Can you work these out from the model? Positions are in its coordinate system, mm. A direction names the side the tool comes from. Round coordinates to 2 decimals unless told otherwise and drop trailing zeros. Order: outer loops, then holes, each group sorted by start corner. A loop starts at its lowest first (then second) coordinate and runs counter-clockwise, first axis right, second up.
from build123d import *

# Parameters (mm, degrees)
SKETCH_1_W          = 21
SKETCH_1_H          = 34
EXTRUDE_1_DEPTH     = 9
SKETCH_4_W          = 21
SKETCH_4_H          = 10
CUT_EXTRUDE_1_DEPTH = 6
SKETCH_5_W          = 21
SKETCH_5_H          = 15
CUT_EXTRUDE_2_DEPTH = 3
SKETCH_6_W          = 13.003696042
SKETCH_6_H          = 17
CUT_EXTRUDE_3_DEPTH = 22.914607001
CUT_EXTRUDE_4_DEPTH = 1.8
CUT_EXTRUDE_5_REACH = 29.178
SKETCH_11_R         = 1.65
HOLE_WIZARD_1_D     = 1.3


with BuildPart() as part:
    # 草图1 → 凸台-拉伸1 (new body)
    with BuildSketch(Plane(origin=(0, 0, 0), x_dir=(1, 0, 0), z_dir=(0, 1, 0))):
        Rectangle(SKETCH_1_W, SKETCH_1_H)
    extrude(amount=EXTRUDE_1_DEPTH)

    # 草图4 → 切除-拉伸1 (cut)
    with BuildSketch(Plane.XZ):
        with Locations((0, -12)):
            Rectangle(SKETCH_4_W, SKETCH_4_H)
    extrude(amount=-CUT_EXTRUDE_1_DEPTH, mode=Mode.SUBTRACT)

    # 草图5 → 切除-拉伸2 (cut)
    with BuildSketch(Plane.XZ):
        with Locations((0, -9.5)):
            Rectangle(SKETCH_5_W, SKETCH_5_H)
    extrude(amount=-CUT_EXTRUDE_2_DEPTH, mode=Mode.SUBTRACT)

    # 草图6 → 切除-拉伸3 (cut, through all)
    with BuildSketch(Plane(origin=(0, 9, 0), x_dir=(1, 0, 0), z_dir=(0, 1, 0))):
        with Locations((0, -8.5)):
            Rectangle(SKETCH_6_W, SKETCH_6_H)
    extrude(amount=-CUT_EXTRUDE_3_DEPTH, mode=Mode.SUBTRACT)

    # 草图9 → M3 六角圆柱头螺钉的柱形沉头孔1 (revolve, cut)
    with BuildSketch(Plane(origin=(10.5, 4.5, 11.5), x_dir=(0, 0, -1), z_dir=(0, 1, 0))):
        Polygon((0, 0), (0, 3.998151979), (1.7, 3.998151979), (1.7, 3.4), (3, 3.4), (3, 0.025), (3.025, 0), align=None)
    revolve(axis=Axis((16.85, 4.5, 11.5), (-1, 0, 0)), mode=Mode.SUBTRACT)

    # 草图10 → 切除-拉伸4 (cut)
    with BuildSketch(Plane.ZY.offset(10.5)):
        Polygon((13.174315781, 1.6), (14.848631561, 4.5), (13.174315781, 7.4), (9.825684219, 7.4), (8.151368439, 4.5), (9.825684219, 1.6), align=None)
    extrude(amount=-CUT_EXTRUDE_4_DEPTH, mode=Mode.SUBTRACT)

    # 草图11 → 切除-拉伸5 (cut, up to next)
    with BuildSketch(Plane.ZY.offset(8.7), mode=Mode.PRIVATE) as cut_extrude_5_sk1:
        with Locations((11.5, 4.5)):
            Circle(SKETCH_11_R)
    cut_extrude_5_tool1 = extrude(cut_extrude_5_sk1.sketch, amount=-CUT_EXTRUDE_5_REACH, mode=Mode.PRIVATE) & part.part
    add(cut_extrude_5_tool1.solids().sort_by_distance((-8.7, 4.5, 11.5))[0], mode=Mode.SUBTRACT)

    # 孔1 (through all)
    with Locations(Plane(origin=(0, 9, 0), x_dir=(1, 0, 0), z_dir=(0, 1, 0))):
        with Locations((-7.5, 4.5), (7.5, 4.5)):
            Hole(HOLE_WIZARD_1_D / 2)


solid = part.part
(1) I want a section at B-B, the plane z = 11.5. List the corners of the cut face in (x, y) for me (3 decimals).
(2) I want a section at D-D, the plane z = -4.5. List the corners of the cut face in (x, y) for me.
(3) I want a section at A-A, the plane x = 7.5. List the corners of the cut face in (y, z) for me.
(4) On a 3-axis mill with a long thin cutter (end or side, diameter ignored), from which of +Z, -Z, +X, -X, +Y, -Y can I reach the whole of each face in a straight line? I mean faces 1 (the face through (6.502, 5, 9)), 2 (the face through (0, 1, -2)), 3 (the face through (-10, 1.6, 11)). Say none if no direction works.
(5) If we mould it in two halves opening along Z, with no side actions, what happens to faces 4 (the face through (0, 9, -4)), 5 (the face through (8, 4, 17)), 6 (the face through (6.81, 5.15, 9.93))? For each: pulls with the +Z half, pulls with the -Z half, needs draft (parallel to the pull), parting line crosses it, or undercut.
(6) I want a section at C-C, the plane z = 3. List the corners of the cut face in (x, y) for me.
(7) I'm going to push flat-ended pins straight in: pin 1 Ø2.5 at (y, z) = (4.5, 11.5) entering from -X; pin 2 Ø3 at (y, z) = (3.5, 12) entering from +X; pin 3 Ø2.5 at (x, y) = (-1, 1.5) entering from -Z; pin 4 Ø4.5 at (x, y) = (2.5, 5) entering from +Z. Where does each tip first touch, or does it pass through?
(8) Please list where these lines run through material, in increasing order: probe 1 along X at (y, z) = (7.4, -4.5); probe 2 along X at (y, z) = (8.75, 2); probe 3 along Z at (x, y) = (-7.5, 7.2).
Ans:
1. outline: (-10.5, 0) - (-6.502, 0) - (-6.502, 2.85) - (-8.7, 2.85) - (-8.7, 1.6) - (-10.5, 1.6) - close; (-10.5, 7.4) - (-8.7, 7.4) - (-8.7, 6.15) - (-6.502, 6.15) - (-6.502, 9) - (-10.5, 9) - close; (6.502, 0) - (10.5, 0) - (10.5, 1.475) - (10.475, 1.5) - (7.1, 1.5) - (7.1, 2.8) - (6.502, 2.8) - close; (6.502, 6.2) - (7.1, 6.2) - (7.1, 7.5) - (10.475, 7.5) - (10.5, 7.525) - (10.5, 9) - (6.502, 9) - close
2. outline: (-10.5, 3) - (-8.15, 3) - (-8.15, 9) - (-10.5, 9) - close; (-6.85, 3) - (6.85, 3) - (6.85, 9) - (-6.85, 9) - close; (8.15, 3) - (10.5, 3) - (10.5, 9) - (8.15, 9) - close
3. outline: (0, -2) - (3, -2) - (3, -3.85) - (9, -3.85) - (9, 17) - (0, 17) - close; (3, -7) - (6, -7) - (6, -17) - (9, -17) - (9, -5.15) - (3, -5.15) - close; hole circle Ø6 at (4.5, 11.5)
4. face 1: +Z, +Y, -Y
4. face 2: -Z, +X, -X, -Y
4. face 3: -X
5. face 4: needs draft
5. face 5: pulls with the +Z half
5. face 6: undercut
6. outline: (-10.5, 0) - (-6.5, 0) - (-6.5, 9) - (-10.5, 9) - close; (6.5, 0) - (10.5, 0) - (10.5, 9) - (6.5, 9) - close
7. pin 1: passes through
7. pin 2: stops at x = 7.1
7. pin 3: stops at z = -2
7. pin 4: stops at z = 0
8. probe 1: x = -10.5 to -8.15, -6.85 to 6.85, 8.15 to 10.5
8. probe 2: x = -10.5 to -6.5, 6.5 to 10.5
8. probe 3: z = -17 to -5.15, -3.85 to 17
